Autodesk Inventor part; units mm, degrees
ref_plane "YZ Plane" through (0, 0, 0) normal (1, 0, 0) x (0, 1, 0)
ref_plane "XZ Plane" through (0, 0, 0) normal (0, 1, 0) x (-1, 0, 0)
ref_plane "XY Plane" through (0, 0, 0) normal (0, 0, 1) x (1, 0, 0)
sketch "Skizze1" plane through (0, 0, 0) normal (0, 0, 1) x (1, 0, 0)
  circle A0 centre (0, 0) radius 25
  dimension "d0" = 50
extrude "Extrusion1" add sketch "Skizze1" along normal blind 5
sketch "Skizze2" plane through (0, 0, 5) normal (0, 0, 1) x (1, 0, 0)
  circle A0 centre (0, 0) radius 20
  dimension "d3" = 40
extrude "Extrusion2" add sketch "Skizze2" along normal blind 30
thread "Gewinde1"
chamfer "Fase1" distance 2 angle 45 2 edges at (-20, 0, 35) (-25, 0, 0)
sketch "Skizze3" plane through (0, 0, 0) normal (0, 0, -1) x (-1, 0, 0)
  line L0 (-15, -4) -> (15, -4)
  line L1 (15, -4) -> (15, 4)
  line L2 (15, 4) -> (-15, 4)
  line L3 (-15, 4) -> (-15, -4)
  line L4 (-15, -4) -> (15, 4) construction
  line L5 (15, -4) -> (-15, 4) construction
  line L6 (-4, -15) -> (4, -15)
  line L7 (4, -15) -> (4, 15)
  line L8 (4, 15) -> (-4, 15)
  line L9 (-4, 15) -> (-4, -15)
  line L10 (-4, -15) -> (4, 15) construction
  line L11 (4, -15) -> (-4, 15) construction
  point P0 (0, 0)
  dimension "d11" = 30
  dimension "d12" = 30
  dimension "d13" = 8
  dimension "d14" = 8
extrude "Extrusion3" cut sketch "Skizze3" against normal blind 8
fillet "Rundung1" radius 2 12 edges at (-4, 9.5, 0) (0, 15, 0) (4, 9.5, 0) (9.5, 4, 0) (15, 0, 0) (9.5, -4, 0) (4, -9.5, 0) (-4, -9.5, 0) (0, -15, 0) (-9.5, -4, 0) (-15, 0, 0) (-9.5, 4, 0)
sketch "Skizze4" plane through (0, 0, 5) normal (0, 0, 1) x (1, 0, 0)
  circle A0 centre (0, 0) radius 25.5
  dimension "d18" = 51
extrude "Extrusion4" add sketch "Skizze4" along normal blind 2
properties part number "Flutschraube"
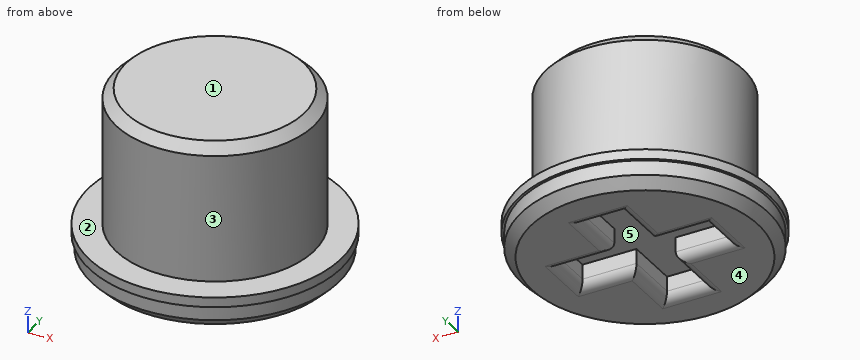
Geometry: final body of the model. Coordinates: model frame, mm. Face numbers are marked on the shaded views. A direction names the side the tool comes from. Give positions to 0.01 mm unless a question says otherwise; leave off trailing zeros. Write each loop counter-clockwise with the first axis right and the second up, starting at its lowest first coordinate (ties: lowest second). Pieces come first, ordered by that corner, then holes.
1. Draft query along X for the marked faces 3, 4 and 5. Return one class per face: released by +X, released by -X, zero draft, split by the parting line, or undercut.
2. Section query C-C, the plane z = 11.5. Return loops of the section in (x, y).
3. Pin query (flat end, axial travel): P1, Ø3, axis at x = -20, z = 28.5, coming from the -Y side; P2, Ø3.5, axis at x = -8.5, z = 3, coming from the +Y side; P3, Ø0.9, axis at y = -8, z = 4, coming from the -X side. Return the tip coordinate at first contact, or that it passes through.
4. Line query: probe 1 along Z at (x, y) = (-5, -2.5); probe 2 along Y at (x, z) = (-13, 7.5); probe 3 along Z at (x, y) = (-21, -8). Output: solid intervals per line, ascending.
5. Reachability of the marked faces 1 and 2 from +Z, -Z, +X, -X, +Y, -Y: full face, straight path, thin tool, end or side. Return the list, or none.
Computed:
1. face 3: split by the parting line
1. face 4: zero draft
1. face 5: undercut
2. outline: circle Ø40 at (0, 0)
3. P1: stops at y = -7.6
3. P2: stops at y = 24.07
3. P3: stops at x = -23.83
4. probe 1: z = 5 to 7, 8 to 35
4. probe 2: y = -15.2 to -4, 4 to 15.2
4. probe 3: z = 0 to 7
5. face 1: +Z, +X, -X, +Y, -Y
5. face 2: +Z
